```python
from build123d import *

# Parameters (mm, degrees)
SKETCH9_W           = 116
SKETCH9_H           = 185
SKETCH9_RX          = 2.0001
SKETCH9_RY          = 2
SKETCH9_W_2         = 14.0398
SKETCH9_H_2         = 76.0678
SKETCH9_W_3         = 8.0434
SKETCH9_H_3         = 14.7638
SKETCH9_W_4         = 9.3662
SKETCH9_H_4         = 16.0866
BOSS_EXTRUDE3_DEPTH = 5


with BuildPart() as part:
    # Sketch9 → Boss-Extrude3 (new body)
    with BuildSketch(Plane.XY):
        with Locations((75.4236, -0.0411)):
            Rectangle(SKETCH9_W, SKETCH9_H)
        with Locations((26.4237, 83.4589)):
            Ellipse(SKETCH9_RX, SKETCH9_RY, mode=Mode.SUBTRACT)
        with Locations((124.4237, 83.4589)):
            Ellipse(SKETCH9_RX, SKETCH9_RY, mode=Mode.SUBTRACT)
        with Locations((124.4237, -83.5411)):
            Ellipse(SKETCH9_RX, SKETCH9_RY, mode=Mode.SUBTRACT)
        with Locations((26.4237, -83.5411)):
            Ellipse(SKETCH9_RX, SKETCH9_RY, mode=Mode.SUBTRACT)
        with Locations((114.1237, 17.1372)):
            Rectangle(SKETCH9_W_2, SKETCH9_H_2, mode=Mode.SUBTRACT)
        with Locations((100.4225, 55.0986)):
            Rectangle(SKETCH9_W_3, SKETCH9_H_3, mode=Mode.SUBTRACT)
        Polygon((88.7925, 30.7834), (104.4559, 30.7834), (104.4559, 16.0196), (104.4559, -13.2439), (96.1886, -13.2439), (96.1886, -28.708), (96.1886, -48.708), (59.0411, -48.708), (59.0411, -28.708), (59.0411, 16.6008), (70.4989, 16.6008), (70.4989, 27.8192), (61.1857, 27.8192), (61.1857, 28.9577), (61.1857, 36.8241), (49.7696, 36.8241), (49.7696, 77.3371), (80.7576, 77.3371), (91.6664, 77.3371), (121.1436, 77.3371), (121.1436, 63.8829), (91.6664, 63.8829), (91.6664, 59.2791), (80.7576, 59.2791), (80.7576, 36.8241), (81.982, 36.8241), (81.982, 28.9577), (81.982, 27.8192), (78.4893, 27.8192), (78.4893, 16.6008), (88.7925, 16.6008), align=None, mode=Mode.SUBTRACT)
        with Locations((41.6049, 47.2397)):
            Rectangle(SKETCH9_W_4, SKETCH9_H_4, mode=Mode.SUBTRACT)
    extrude(amount=BOSS_EXTRUDE3_DEPTH)


solid = part.part
```
The model under review builds one solid part; all positions refer to its coordinate system, in mm. A direction names the side the tool comes from. Round coordinates to 2 decimals unless told otherwise and drop trailing zeros. Loops run counter-clockwise (first coordinate to the right, second up) from the corner with the lowest first, then second, coordinate; pieces in that order, holes last.
Item 1: Take a section at A-A (y = -30). Write out the cut boundary in (x, z), then the cut area to 3 significant figures.
Determined:
outline: (17.42, 0) - (59.04, 0) - (59.04, 5) - (17.42, 5) - close; (96.19, 0) - (133.42, 0) - (133.42, 5) - (96.19, 5) - close
area: 394 mm2
Item 2: Take a section at B-B (x = 102). Write out the cut boundary in (y, z).
Determined:
outline: (-92.54, 0) - (-13.24, 0) - (-13.24, 5) - (-92.54, 5) - close; (30.78, 0) - (47.72, 0) - (47.72, 5) - (30.78, 5) - close; (62.48, 0) - (63.88, 0) - (63.88, 5) - (62.48, 5) - close; (77.34, 0) - (92.46, 0) - (92.46, 5) - (77.34, 5) - close
Item 3: Take a section at C-C (x = 63). Write out the cut boundary in (y, z).
Determined:
outline: (-92.54, 0) - (-48.71, 0) - (-48.71, 5) - (-92.54, 5) - close; (16.6, 0) - (27.82, 0) - (27.82, 5) - (16.6, 5) - close; (77.34, 0) - (92.46, 0) - (92.46, 5) - (77.34, 5) - close
Item 4: Mouldability with a two-part tool opening along X and no side actions: class faces 1 (the face through (84, 16.601, 2)), 2 (the face through (75, 92.459, 2)) as released by +X, released by -X, zero draft, split by the parting line, or undercut.
Determined:
face 1: undercut
face 2: zero draft
Item 5: For line 1 (X direction, y = -17, z = 4.2); line 2 (Y direction, x = 64, z = 4.35); line 3 (Y direction, x = 112, z = 2.1), list the stretches that pass through material, from the lowest coordinate up.
Determined:
line 1: x = 17.42 to 59.04, 96.19 to 107.1, 121.14 to 133.42
line 2: y = -92.54 to -48.71, 16.6 to 27.82, 77.34 to 92.46
line 3: y = -92.54 to -20.9, 55.17 to 63.88, 77.34 to 92.46
Item 6: Take a section at D-D (y = -10.5). Write out the cut boundary in (x, z), then the cut area to 3 significant figures.
Determined:
outline: (17.42, 0) - (59.04, 0) - (59.04, 5) - (17.42, 5) - close; (104.46, 0) - (107.1, 0) - (107.1, 5) - (104.46, 5) - close; (121.14, 0) - (133.42, 0) - (133.42, 5) - (121.14, 5) - close
area: 283 mm2
Item 7: Clearance check with a flat-ended pin moving along its axis: pin 1 Ø2 at (x, y) = (44, -66) entering from -Z. State where the tip first meets the part, or that it passes through.
Determined:
pin 1: stops at z = 0
Item 8: For faces 3 (the face through (49, 1, 5)), 4 (the face through (80, 27.819, 2)), list the 3-axis set-ups (+Z, -Z, +X, -X, +Y, -Y) from which the entire face can be reached by the end or side of a thin tool; tool diameter is ignored.
Determined:
face 3: +Z, +X, -X, +Y, -Y
face 4: +Z, -Z
